```python
from build123d import *

# Parameters (mm, degrees)
F0_W      = 420
F0_H      = 420
F1_DEPTH  = 105
F2_T      = -6
F3_W      = 6
F3_H      = 408
F4_DEPTH  = 18
F5_W      = 6
F5_H      = 408
F6_DEPTH  = 18
F7_W      = 6
F7_H      = 18
F8_DEPTH  = 372
F9_W      = 6
F9_H      = 18
F10_DEPTH = 372
F11_W     = 408
F11_H     = 408
F11_W_2   = 400
F11_H_2   = 400
F12_DEPTH = 10
F14_DEPTH = 25.4
F15_W     = 400
F15_H     = 400
F16_DEPTH = 10
F18_DEPTH = 25.4


with BuildPart() as f1:
    # F0 (on Front) → F1 (new body, symmetric)
    with BuildSketch(Plane.XZ):
        Rectangle(F0_W, F0_H)
    extrude(amount=F1_DEPTH, both=True)

    # F2
    f2_openings = [f1.faces().sort_by_distance(p)[0] for p in [
        (0, -105, 0),
    ]]
    offset(amount=F2_T, openings=f2_openings)

    # F3 (on face) → F4 (join)
    with BuildSketch(Plane.YZ.offset(-204)):
        with Locations((-92, 0)):
            Rectangle(F3_W, F3_H)
    extrude(amount=F4_DEPTH)

    # F5 (on face) → F6 (join)
    with BuildSketch(Plane(origin=(204, 0, 0), x_dir=(0, -1, 0), z_dir=(-1, 0, 0))):
        with Locations((92, 0)):
            Rectangle(F5_W, F5_H)
    extrude(amount=F6_DEPTH)

    # F7 (on face) → F8 (join, through all)
    with BuildSketch(Plane.YZ.offset(-186)):
        with Locations((-92, 195)):
            Rectangle(F7_W, F7_H)
    extrude(amount=F8_DEPTH)

    # F9 (on face) → F10 (join, through all)
    with BuildSketch(Plane.YZ.offset(-186)):
        with Locations((-92, -195)):
            Rectangle(F9_W, F9_H)
    extrude(amount=F10_DEPTH)

    # F11 (on face) → F12 (join)
    with BuildSketch(Plane.XZ.offset(95)):
        Rectangle(F11_W, F11_H)
        Rectangle(F11_W_2, F11_H_2, mode=Mode.SUBTRACT)
    extrude(amount=F12_DEPTH)

    # F13: F1 across face


with BuildPart() as f1_1:
    add(f1.part)
    add(f1.part.mirror(Plane(origin=(0, 105, 0), x_dir=(1, 0, 0), z_dir=(0, 1, 0))))

    # F14 (cut): a face of the model
    f14_faces = [f1_1.faces().sort_by_distance(p)[0] for p in [
        (0, 111, 0),
    ]]
    extrude(f14_faces, amount=-F14_DEPTH, mode=Mode.SUBTRACT)

    # F15 (on face) → F16 (join)
    with BuildSketch(Plane(origin=(0, 305, 0), x_dir=(-1, 0, 0), z_dir=(0, 1, 0))):
        Rectangle(F15_W, F15_H)
    extrude(amount=F16_DEPTH)

    # F17: F1 across face


with BuildPart() as f1_2:
    add(f1_1.part)
    add(f1_1.part.mirror(Plane(origin=(204, 105, 0), x_dir=(0, -1, 0), z_dir=(-1, 0, 0))))

    # F18 (cut): a face of the model
    f18_faces = [f1_2.faces().sort_by_distance(p)[0] for p in [
        (198, 105, 0),
    ]]
    extrude(f18_faces, amount=-F18_DEPTH, mode=Mode.SUBTRACT)


solid = f1_2.part
```
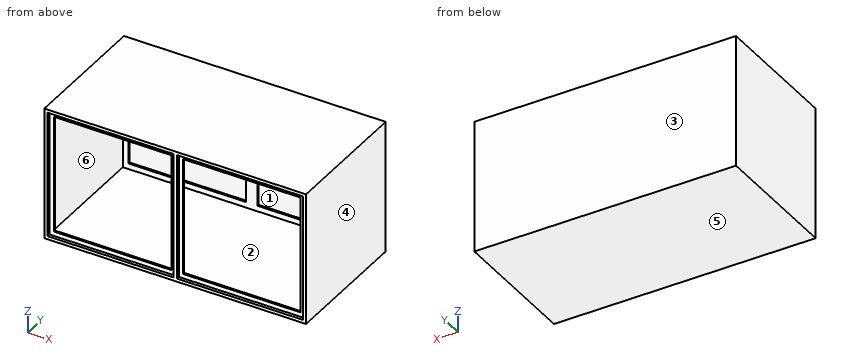
Work out the finished part from the listing and answer in its coordinate system (mm). Face numbers are marked on the shaded views. A direction names the side the tool comes from. Coordinates: 2 decimals unless noted, no trailing zeros. Write each loop counter-clockwise with the first axis right and the second up, starting at its lowest first coordinate (ties: lowest second). Pieces come first, ordered by that corner, then holes.
Q1. A cutting plane is placed at B-B, the plane y = -12. Give the vertices of the cut face in (x, z), then the cut area to 3 significant figures.
Q2. Determine the mould class of the marked faces 4, 5 and 6 for opening direction Z: released by +Z, released by -Z, zero draft, split by the parting line, or undercut.
Q3. Which of the six approach directions +Z, -Z, +X, -X, +Y, -Y give full straight-line access (tool end or side, diameter ignored) to the marked faces 1, 2 and 3?
Q4. Find the intervals of material crossed by line 1 (X direction, y = -83, z = 38.5); line 2 (Z direction, x = 126.5, y = 268); line 3 (Y direction, x = 306, z = -67), in increasing order.
Q5. A cutting plane is placed at C-C, the plane x = -127.5. Give the vertices of the cut face in (y, z), then the cut area to 3 significant figures.
Findings below:
1. outline: (-210, -210) - (618, -210) - (618, 210) - (-210, 210) - close; hole (-204, -204) - (612, -204) - (612, 204) - (-204, 204) - close
1. area: 14,800 mm2
2. face 4: zero draft
2. face 5: released by -Z
2. face 6: undercut
3. face 1: -Y
3. face 2: none
3. face 3: +Z, -Z, +X, -X, +Y
4. line 1: x = -210 to -204, 612 to 618
4. line 2: z = -210 to -204, 204 to 210
4. line 3: y = 305 to 315
5. outline: (-105, -210) - (315, -210) - (315, 210) - (-105, 210) - (-105, 200) - (-95, 200) - (-95, 186) - (-89, 186) - (-89, 204) - (299, 204) - (299, 186) - (305, 186) - (305, -186) - (299, -186) - (299, -204) - (-89, -204) - (-89, -186) - (-95, -186) - (-95, -200) - (-105, -200) - close
5. area: 9,630 mm2
